```python
from build123d import *

# Parameters (mm, degrees)
CROQUIS1_W              = 40
CROQUIS1_H              = 40
SALIENTE_EXTRUIR1_DEPTH = 119.15
CROQUIS2_R              = 10.4
SALIENTE_EXTRUIR2_DEPTH = 3.4
SALIENTE_EXTRUIR3_DEPTH = 1.27
CROQUIS4_R              = 2.5
CORTAR_EXTRUIR1_DEPTH   = 5
CROQUIS5_W              = 9
CROQUIS5_H              = 6
CORTAR_EXTRUIR2_DEPTH   = 9
CROQUIS6_R              = 1.5
CORTAR_EXTRUIR3_DEPTH   = 3.5
SALIENTE_EXTRUIR4_DEPTH = 8
CROQUIS10_W             = 0.2
CROQUIS10_H             = 40
CORTAR_EXTRUIR4_DEPTH   = 0.2
MATRIZC1_COUNT          = 4


with BuildPart() as part:
    # Croquis1 → Saliente-Extruir1 (new body)
    with BuildSketch(Plane.XY):
        Rectangle(CROQUIS1_W, CROQUIS1_H)
    extrude(amount=-SALIENTE_EXTRUIR1_DEPTH)

    # Croquis2 → Saliente-Extruir2 (add)
    with BuildSketch(Plane.XY):
        Circle(CROQUIS2_R)
    extrude(amount=SALIENTE_EXTRUIR2_DEPTH)

    # Croquis3 → Saliente-Extruir3 (add)
    with BuildSketch(Plane.XY):
        with BuildLine():
            Line((-16, 13.1), (-16, 16))
            Line((-16, 16), (-13.1, 16))
            ThreePointArc((-13.1, 16), (-18.050609665, 18.050609665), (-16, 13.1))
        make_face()
        with BuildLine():
            Line((-13.1, 16), (-16, 16))
            Line((-16, 16), (-16, 13.1))
            ThreePointArc((-16, 13.1), (-13.949390335, 13.949390335), (-13.1, 16))
        make_face()
        with BuildLine():
            ThreePointArc((18.9, 16), (16, 18.9), (13.1, 16))
            Line((13.1, 16), (16, 16))
            Line((16, 16), (16, 13.1))
            ThreePointArc((16, 13.1), (18.050609665, 13.949390335), (18.9, 16))
        make_face()
        with BuildLine():
            Line((16, 16), (13.1, 16))
            ThreePointArc((13.1, 16), (13.949390335, 13.949390335), (16, 13.1))
            Line((16, 13.1), (16, 16))
        make_face()
        with BuildLine():
            ThreePointArc((-13.1, -16), (-13.949390335, -13.949390335), (-16, -13.1))
            Line((-16, -13.1), (-16, -16))
            Line((-16, -16), (-13.1, -16))
        make_face()
        with BuildLine():
            Line((-16, -16), (-16, -13.1))
            ThreePointArc((-16, -13.1), (-18.050609665, -18.050609665), (-13.1, -16))
            Line((-13.1, -16), (-16, -16))
        make_face()
        with BuildLine():
            ThreePointArc((18.9, -16), (18.050609665, -13.949390335), (16, -13.1))
            Line((16, -13.1), (16, -16))
            Line((16, -16), (13.1, -16))
            ThreePointArc((13.1, -16), (16, -18.9), (18.9, -16))
        make_face()
        with BuildLine():
            Line((16, -16), (16, -13.1))
            ThreePointArc((16, -13.1), (13.949390335, -13.949390335), (13.1, -16))
            Line((13.1, -16), (16, -16))
        make_face()
    extrude(amount=SALIENTE_EXTRUIR3_DEPTH)

    # Croquis4 → Cortar-Extruir1 (cut)
    with BuildSketch(Plane.XY.offset(3.4)):
        Circle(CROQUIS4_R)
    extrude(amount=-CORTAR_EXTRUIR1_DEPTH, mode=Mode.SUBTRACT)

    # Croquis5 → Cortar-Extruir2 (cut)
    with BuildSketch(Plane(origin=(0, 0, -119.15), x_dir=(-1, 0, 0), z_dir=(0, 0, -1))):
        with Locations((0, -17)):
            Rectangle(CROQUIS5_W, CROQUIS5_H)
    extrude(amount=-CORTAR_EXTRUIR2_DEPTH, mode=Mode.SUBTRACT)

    # Croquis6 → Cortar-Extruir3 (cut)
    with BuildSketch(Plane(origin=(20, 0, 0), x_dir=(0, 0, -1), z_dir=(1, 0, 0))):
        with Locations(Location((38, 0, 0), (0, 0, 90))):
            Circle(CROQUIS6_R)
        with Locations(Location((8.5, 0, 0), (0, 0, 90))):
            Circle(CROQUIS6_R)
        with Locations(Location((63.5, 0, 0), (0, 0, 90))):
            Circle(CROQUIS6_R)
        with Locations(Location((12, 8, 0), (0, 0, 90))):
            Circle(CROQUIS6_R)
        with Locations(Location((12, -8, 0), (0, 0, 90))):
            Circle(CROQUIS6_R)
        with Locations(Location((8.5, -10, 0), (0, 0, 90))):
            Circle(CROQUIS6_R)
        with Locations(Location((8.5, 10, 0), (0, 0, 90))):
            Circle(CROQUIS6_R)
        with Locations(Location((67, -7.75, 0), (0, 0, 90))):
            Circle(CROQUIS6_R)
        with Locations(Location((63.5, -15.5, 0), (0, 0, 90))):
            Circle(CROQUIS6_R)
        with Locations(Location((67, 7.75, 0), (0, 0, 90))):
            Circle(CROQUIS6_R)
        with Locations(Location((63.5, 15.5, 0), (0, 0, 90))):
            Circle(CROQUIS6_R)
    extrude(amount=-CORTAR_EXTRUIR3_DEPTH, mode=Mode.SUBTRACT)

    # Croquis9 → Saliente-Extruir4 (add)
    with BuildSketch(Plane(origin=(0, 0, -119.15), x_dir=(-1, 0, 0), z_dir=(0, 0, -1))):
        Polygon((-6.829794284, -20), (-6.829794284, -11.650544172), (6.829794284, -11.650544172), (6.829794284, -20), (4.5, -20), (4.5, -14), (-4.5, -14), (-4.5, -20), align=None)
    extrude(amount=SALIENTE_EXTRUIR4_DEPTH)

    # Croquis10 → Cortar-Extruir4 (cut)
    with BuildSketch(Plane(origin=(20, 0, 0), x_dir=(0, 0, -1), z_dir=(1, 0, 0))):
        with Locations((73, 0)):
            Rectangle(CROQUIS10_W, CROQUIS10_H)
        with Locations((2.5, 0)):
            Rectangle(CROQUIS10_W, CROQUIS10_H)
    cortar_extruir4 = extrude(amount=-CORTAR_EXTRUIR4_DEPTH, mode=Mode.SUBTRACT)

    # MatrizC1: Cortar-Extruir4 ×4 about axis
    matrizc1_axis = Axis((0, 0, 0), (0, 0, 1))
    for i in range(1, MATRIZC1_COUNT):
        add(cortar_extruir4.rotate(matrizc1_axis, i * 360 / MATRIZC1_COUNT), mode=Mode.SUBTRACT)


solid = part.part
```
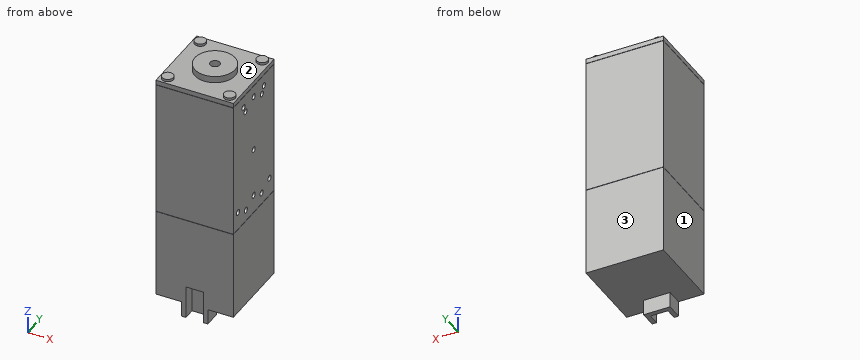
Model file for the job. Use its own axes, mm. Face numbers are marked on the shaded views. Coordinates: 2 decimals unless noted, no trailing zeros. Order: outer loops, then holes, each group sorted by start corner. A loop starts at its lowest first (then second) coordinate and runs counter-clockwise, first axis right, second up. Notation, with made-up numbers: (-2, 74) - (54, 74) arc R9 cw to (54, 90) - close; hole circle Ø4 at (56, -4). An arc over 180 degrees is marked (long way). Return JSON: item names as keys, results as strings. Group by question number.
1) Mould opens along X. For the marked faces 1, 2 and 3 say: released by +X, released by -X, zero draft, split by the parting line, or undercut.
2) Probe line 1 (Y direction, x = 18.75, z = -67); line 2 (Z direction, x = 18.5, y = 8); line 3 (Z direction, x = 18, y = 0). List the from-to ranges inside material, lowest first. Write a range as from..to.
3) Flat gauge pins, fed straight in: P1, Ø1.8, axis at y = -10, z = -8.5, coming from the +X side; P2, Ø2.5, axis at x = -1.5, z = -114.5, coming from the -Y side; P3, Ø6, axis at x = -10.5, y = 9.5, coming from the -Z side. Where does each tip first touch, or does it go through?
4) Saw through at A-A, the plane z = -8.5. Write the cut outline in (x, y).
5) Saw through at B-B, the plane x = 8.5. Write the cut outline in (y, z).
Values found:
{
 "1": {"face 1": "released by -X", "face 2": "undercut", "face 3": "zero draft"},
 "2": {"line 1": "y = -20..-9.25, -6.25..6.25, 9.25..20", "line 2": "z = -119.15..-68.48, -65.52..-13.5, -10.5..0", "line 3": "z = -119.15..-65, -62..-39.5, -36.5..-10, -7..0"},
 "3": {"P1": "stops at x = 16.5", "P2": "stops at y = -14", "P3": "stops at z = -119.15"},
 "4": {"outline": "(-20, -20) - (20, -20) - (20, -11.5) - (16.5, -11.5) - (16.5, -8.5) - (20, -8.5) - (20, -1.5) - (16.5, -1.5) - (16.5, 1.5) - (20, 1.5) - (20, 8.5) - (16.5, 8.5) - (16.5, 11.5) - (20, 11.5) - (20, 20) - (-20, 20) - close"},
 "5": {"outline": "(-20, -119.15) - (20, -119.15) - (20, -73.1) - (19.8, -73.1) - (19.8, -72.9) - (20, -72.9) - (20, -2.6) - (19.8, -2.6) - (19.8, -2.4) - (20, -2.4) - (20, 0) - (5.99, 0) - (5.99, 3.4) - (-5.99, 3.4) - (-5.99, 0) - (-20, 0) - (-20, -2.4) - (-19.8, -2.4) - (-19.8, -2.6) - (-20, -2.6) - (-20, -72.9) - (-19.8, -72.9) - (-19.8, -73.1) - (-20, -73.1) - close"}
}
